Check sheet for the modelled part. Datum: model origin and axes. Units: mm. Face numbers are marked on the shaded views. A direction names the side the tool comes from. Round coordinates to 2 decimals unless told otherwise and drop trailing zeros. Write each loop counter-clockwise with the first axis right and the second up, starting at its lowest first coordinate (ties: lowest second). Pieces come first, ordered by that corner, then holes. Notation, with made-up numbers: (17, 74) -> (43, 74) arc R17 cw to (43, 85) -> close; hole circle Ø10 at (77.25, 47). An arc over 180 degrees is marked (long way). Write item = value, one per line.
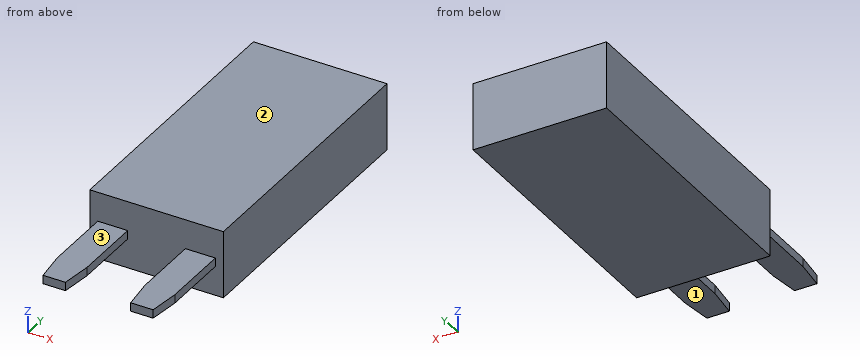
from build123d import *

# Parameters (mm, degrees)
SKETCH1_W             = 12.5
SKETCH1_H             = 26
BOSS_EXTRUDE1_DEPTH   = 3.15
SKETCH2_W             = 2.8
SKETCH2_H             = 0.8
BOSS_EXTRUDE2_DEPTH   = 9.3
CHAMFER1_SIZE         = 0.35
CHAMFER1_SIZE2        = 2.85052125
CHAMFER1_PART_2_SIZE  = 0.35
CHAMFER1_PART_2_SIZE2 = 2.85052125


with BuildPart() as part:
    # Sketch1 → Boss-Extrude1 (new body, symmetric)
    with BuildSketch(Plane.XY):
        Rectangle(SKETCH1_W, SKETCH1_H)
    extrude(amount=BOSS_EXTRUDE1_DEPTH, both=True)

    # Sketch2 → Boss-Extrude2 (add)
    with BuildSketch(Plane.XZ.offset(13)):
        with Locations((4.1, 0)):
            Rectangle(SKETCH2_W, SKETCH2_H)
        with Locations((-4.1, 0)):
            Rectangle(SKETCH2_W, SKETCH2_H)
    extrude(amount=BOSS_EXTRUDE2_DEPTH)

    # Chamfer1
    chamfer1_edges = [part.edges().sort_by_distance(p)[0] for p in [
        (-5.5, -22.3, 0),
        (-2.7, -22.3, 0),
    ]]
    chamfer1_side = [part.faces().sort_by_distance(p)[0] for p in [
        (-4.1, -22.3, 0),
    ]]
    chamfer(chamfer1_edges, length=CHAMFER1_SIZE, length2=CHAMFER1_SIZE2, reference=chamfer1_side[0])

    # Chamfer1 part 2
    chamfer1_part_2_edges = [part.edges().sort_by_distance(p)[0] for p in [
        (2.7, -22.3, 0),
        (5.5, -22.3, 0),
    ]]
    chamfer1_part_2_side = [part.faces().sort_by_distance(p)[0] for p in [
        (4.1, -22.3, 0),
    ]]
    chamfer(chamfer1_part_2_edges, length=CHAMFER1_PART_2_SIZE, length2=CHAMFER1_PART_2_SIZE2, reference=chamfer1_part_2_side[0])


solid = part.part
(1) Sectioned sample at A-A on y = -15.5. Enter the section's corners in (x, z), then the cut area to 3 significant figures.
Worked answers:
outline = (-5.5, -0.4) -> (-2.7, -0.4) -> (-2.7, 0.4) -> (-5.5, 0.4) -> close; (2.7, -0.4) -> (5.5, -0.4) -> (5.5, 0.4) -> (2.7, 0.4) -> close
area = 4.48 mm²
(2) Access from +Z, -Z, +X, -X, +Y, -Y to the whole of each face (thin tool, end or side, straight path). Record for the marked faces 1, 2 and 3.
Worked answers:
face_1 = -Z, +X, -X, -Y
face_2 = +Z, +X, -X, +Y, -Y
face_3 = +Z, +X, -X, -Y
(3) Sectioned sample at B-B on z = -2.5. Enter the section's corners in (x, y).
Worked answers:
outline = (-6.25, -13) -> (6.25, -13) -> (6.25, 13) -> (-6.25, 13) -> close
(4) Sectioned sample at C-C on x = -0.25. Enter the section's corners in (y, z).
Worked answers:
outline = (-13, -3.15) -> (13, -3.15) -> (13, 3.15) -> (-13, 3.15) -> close
(5) Go/stop test with flat-tipped pins: P1, Ø3, axis at x = 3.5, y = -16, coming from the +Z side; P2, Ø2, axis at x = -3.5, y = -16.5, coming from the -Z side; P3, Ø1.9, axis at x = 1.5, z = 1.5, coming from the -Y side. Record where each tip stops, or that it passes through.
Worked answers:
P1 = 0.4
P2 = -0.4
P3 = -13
(6) Material ranges on L1, parallel to Y at x = 5, z = -0.75; L2, parallel to Z at x = 4, y = -15.5, recorded low to high. Write a range as [from, to].
Worked answers:
L1 = [-13, 13]
L2 = [-0.4, 0.4]
